```python
from build123d import *

# Parameters (mm, degrees)
ESQUISSE1_W             = 30
ESQUISSE1_H             = 41
EXTRUSION1_DEPTH        = 16
CONG_1_R                = 15
ESQUISSE3_R             = 4
ENL_V_MAT_EXTRU_1_DEPTH = 2.5
ESQUISSE4_R             = 1
ENL_V_MAT_EXTRU_2_DEPTH = 53.566624392


with BuildPart() as part:
    # Esquisse1 → Extrusion1 (new body)
    with BuildSketch(Plane(origin=(0, 0, 0), x_dir=(1, 0, 0), z_dir=(0, 1, 0))):
        with Locations((15, 20.5)):
            Rectangle(ESQUISSE1_W, ESQUISSE1_H)
    extrude(amount=EXTRUSION1_DEPTH)

    # Congé1
    cong_1_edges = [part.edges().sort_by_distance(p)[0] for p in [
        (30, 8, -41),
        (0, 8, -41),
    ]]
    fillet(cong_1_edges, radius=CONG_1_R - 0.0001)  # a hair under: the kernel refuses the full size

    # Esquisse3 → Enlèv. mat.-Extru.1 (cut)
    with BuildSketch(Plane(origin=(0, 16, 0), x_dir=(1, 0, 0), z_dir=(0, 1, 0))):
        with Locations(Location((15, 26, 0), (0, 0, 270))):
            Circle(ESQUISSE3_R)
    extrude(amount=-ENL_V_MAT_EXTRU_1_DEPTH, mode=Mode.SUBTRACT)

    # Esquisse4 → Enlèv. mat.-Extru.2 (cut, through all)
    with BuildSketch(Plane(origin=(0, 13.5, 0), x_dir=(1, 0, 0), z_dir=(0, 1, 0))):
        with Locations(Location((15, 26, 0), (0, 0, 270))):
            Circle(ESQUISSE4_R)
    extrude(amount=-ENL_V_MAT_EXTRU_2_DEPTH, mode=Mode.SUBTRACT)


solid = part.part
```
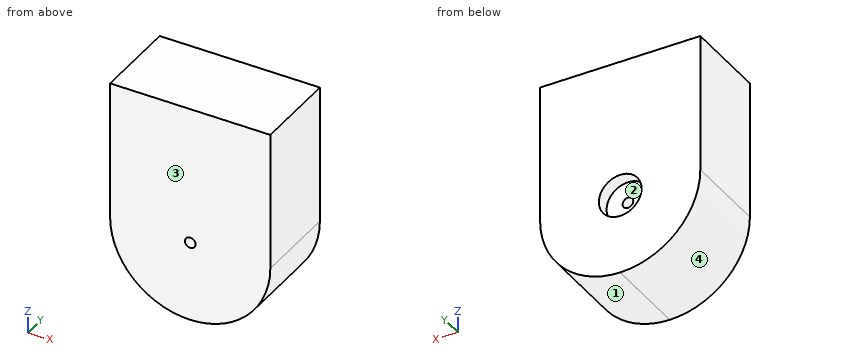
The listing builds one solid part. Answer for the finished solid, in the listing's coordinates (mm). Face numbers are marked on the shaded views. Coordinates: 2 decimals unless noted, no trailing zeros. Loops run counter-clockwise (first coordinate to the right, second up) from the corner with the lowest first, then second, coordinate; pieces in that order, holes last. Notation, with made-up numbers: M 88.5,10 L 120.5,10 A29 cw 120.5,48 Z; hole C 29.5,32.25 d11. An arc over 180 degrees is marked long. Answer as CSV lines item,"result". Start each with the question number.
(1) The part is cut by section D-D (x = 18.5). Give the vertices of the cut face in (y, z), and give its area (3 significant figures).
(2) Find the intervals of material crossed by L1, parallel to X at y = 15.2, z = -26; L2, parallel to X at y = 7.25, z = -26; L3, parallel to Y at x = 13, z = -24, in increasing order. Write a range as [from, to].
(3) Given pin 1 (4 mm diameter, centred on x = 15.5, z = -26, fed in from +Y); pin 2 (1.5 mm diameter, centred on x = 23.5, y = 10.5, fed in from +Z); pin 3 (2 mm diameter, centred on x = 9, y = 3, fed in from -Z); pin 4 (5 mm diameter, centred on x = 11.5, y = 12.5, fed in from -Z), each flat-ended and moving along its own axis, determine where each tip first touches the part or whether it passes through.
(4) The part is cut by section C-C (z = -23.5). Give the vertices of the cut face in (x, y).
(5) The part is cut by section B-B (x = 14.5). Give the vertices of the cut face in (y, z).
(6) The mould has two halves that part along X. Classify the marked faces 1, 2, 3 and 4: pulls with the +X half, pulls with the -X half, needs draft (parallel to the pull), parting line crosses it, or undercut.
Determined:
1,outline,"M 0,-40.59 L 16,-40.59 L 16,-27.94 L 13.5,-27.94 L 13.5,-24.06 L 16,-24.06 L 16,0 L 0,0 Z"
1,area,"640 mm2"
2,L1,"[0, 11], [19, 30]"
2,L2,"[0, 14], [16, 30]"
2,L3,"[0, 13.5]"
3,pin 1,"y = 13.5"
3,pin 2,"z = 0"
3,pin 3,"z = -40.14"
3,pin 4,"z = -40.97"
4,outline,"M 0,0 L 30,0 L 30,16 L 18.12,16 L 18.12,13.5 L 11.88,13.5 L 11.88,16 L 0,16 Z"
5,outline,"M 0,-40.99 L 16,-40.99 L 16,-29.97 L 13.5,-29.97 L 13.5,-26.87 L 0,-26.87 Z; M 0,-25.13 L 13.5,-25.13 L 13.5,-22.03 L 16,-22.03 L 16,0 L 0,0 Z"
6,face 1,"pulls with the +X half"
6,face 2,"undercut"
6,face 3,"needs draft"
6,face 4,"pulls with the -X half"
